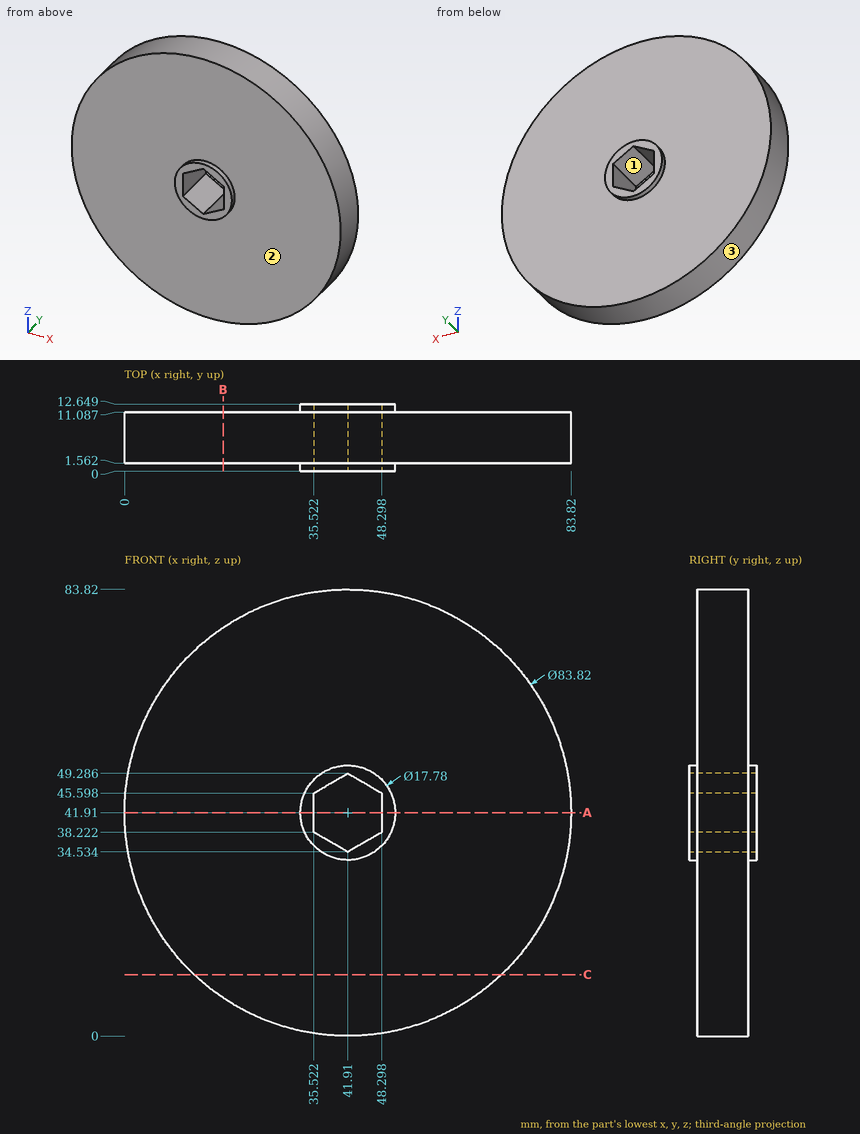
Check sheet for the drawn part. Datum: minimum x, y, z corner. Units: mm. Give positions to 0.01 mm unless a question says otherwise; leave off trailing zeros. Order: outer loops, then holes, each group sorted by start corner. A loop starts at its lowest first (then second) coordinate and runs counter-clockwise, first axis right, second up. Notation, with made-up numbers: (25.5, 12.5) -> (33.5, 12.5) arc R16 cw to (33.5, 33.5) -> close; hole circle Ø1 at (52, -1.75). An arc over 180 degrees is marked (long way). Use a Markdown table: item, result.
1) Section check B-B, the plane x = 18.5. Record the boundary of the cut face in (y, z).
Results:
| item | result |
|---|---|
| outline | (1.56, 7.15) -> (11.09, 7.15) -> (11.09, 76.67) -> (1.56, 76.67) -> close |
2) Material ranges on probe 1 along X at (y, z) = (9.5, 42.5); probe 2 along Y at (x, z) = (59.5, 4); probe 3 along Z at (x, y) = (37, 9.25), recorded low to high.
Results:
| item | result |
|---|---|
| probe 1 | 0 to 35.52, 48.3 to 83.82 |
| probe 2 | 1.56 to 11.09 |
| probe 3 | 0.29 to 37.37, 46.45 to 83.53 |
3) Mould release check, pull along X, two halves, no side actions. Record for the marked faces 1, 2 and 3: pulls with the +X half, pulls with the -X half, needs draft (parallel to the pull), parting line crosses it, or undercut.
Results:
| item | result |
|---|---|
| face 1 | undercut |
| face 2 | needs draft |
| face 3 | parting line crosses it |
4) Depth check by flat-ended pin: pin 1 Ø3 at (x, z) = (55.5, 39.5) entering from -Y; pin 2 Ø5 at (y, z) = (1.5, 11.5) entering from +X (1 decimal); pin 3 Ø3 at (y, z) = (4.5, 66.5) entering from -X (1 decimal). Enter the tip coordinate at first touch or a pass-through.
Results:
| item | result |
|---|---|
| pin 1 | y = 1.56 |
| pin 2 | x = 73.2 |
| pin 3 | x = 6.9 |
5) Section check A-A, the plane z = 41.91. Record the boundary of the cut face in (x, y).
Results:
| item | result |
|---|---|
| outline | (0, 1.56) -> (33.02, 1.56) -> (33.02, 0) -> (35.52, 0) -> (35.52, 12.65) -> (33.02, 12.65) -> (33.02, 11.09) -> (0, 11.09) -> close; (48.3, 0) -> (50.8, 0) -> (50.8, 1.56) -> (83.82, 1.56) -> (83.82, 11.09) -> (50.8, 11.09) -> (50.8, 12.65) -> (48.3, 12.65) -> close |
6) Section check C-C, the plane z = 11.5. Record the boundary of the cut face in (x, y).
Results:
| item | result |
|---|---|
| outline | (13.07, 1.56) -> (70.75, 1.56) -> (70.75, 11.09) -> (13.07, 11.09) -> close |
